Input: part model. Units: mm. Frame: model coordinates. A direction names the side the tool comes from. Round coordinates to 2 decimals unless told otherwise and drop trailing zeros. Order: outer loops, then holes, each group sorted by start corner. A loop starts at its lowest first (then second) coordinate and runs counter-clockwise, first axis right, second up.
Item 1: Reachability of faces 5 (the cylindrical face through (-2.75, 0.36, -12.4)), 6 (the flat face through (-6, -12, -44.45)) from +Z, -Z, +X, -X, +Y, -Y: full face, straight path, thin tool, end or side. Return the list, or none.
Item 2: Mould query, pull axis X, two halves, no side actions, for faces 1 (the flat face through (25.4, 0, -10)), 2 (the flat face through (-25.4, 0, -9)), 3 (the flat face through (-3, -6, -50.8)), 4 (the cylindrical face through (-1.03, -0.36, -20.75)). Classes: released by +X, released by -X, zero draft, split by the parting line, or undercut.
Item 3: Cut plane C-C on y = -7.5. Give the number of separate pieces and of enclosed holes in the cut face, then the cut area to 3 significant figures.
Item 4: Cut plane B-B on x = 8.5. Output: boundary loops of the cut face in (y, z).
Item 5: Cut plane A-A on z = -25.4. Output: boundary loops of the cut face in (x, y).
Item 6: Line query: L1, parallel to Z at x = 0, y = -1; L2, parallel to Z at x = 0, y = 9; L3, parallel to X at y = -10, z = -25. Output: solid intervals per line, ascending.
Item 7: First-contact query: pin 1 (4 mm diameter, centred on x = -1.5, y = 3, fed in from -Z); pin 2 (7.5 mm diameter, centred on x = 0, z = -25.4, fed in from +Y). Flat tips, straight axial feed; report the tip coordinate or a pass-through.
Item 8: Cut plane D-D on z = 0. Output: boundary loops of the cut face in (x, y).
```python
from build123d import *

# Parameters (mm, degrees)
F0_R     = 12.7
F1_DEPTH = 25.4


with BuildPart() as f1:
    # F0 (on Front) → F1 (new body, symmetric)
    with BuildSketch(Plane.XZ):
        Polygon((-12.7, -44.45), (0, -44.45), (12.7, -44.45), (25.4, -44.45), (25.4, 25.4), (-25.4, 25.4), (-25.4, -44.45), align=None)
        with BuildLine():
            ThreePointArc((0, -30.1625), (-3.3675960454, -22.0324039546), (4.7625, -25.4))
            ThreePointArc((4.7625, -25.4), (3.3675960454, -28.7675960454), (0, -30.1625))
        make_face(mode=Mode.SUBTRACT)
        Circle(F0_R, mode=Mode.SUBTRACT)
    extrude(amount=F1_DEPTH, both=True)

    # F0 (on Front) → F2 (revolve)
    with BuildSketch(Plane.XZ):
        Polygon((12.7, -44.45), (0, -44.45), (0, -50.8), (6.35, -50.8), (12.7, -50.8), align=None)
        Polygon((6.35, -50.8), (0, -50.8), (0, -53.34), (2.54, -53.34), (6.35, -53.34), align=None)
        Polygon((2.54, -53.34), (0, -53.34), (0, -57.15), align=None)
    revolve(axis=Axis((0, 0, -41.275), (0, 0, -1)))


solid = f1.part
```
From the geometry:
1. face 5: +Y, -Y
1. face 6: -Z
2. face 1: released by +X
2. face 2: released by -X
2. face 3: zero draft
2. face 4: undercut
3. separate pieces: 1
3. enclosed holes: 2
3. area: 3,100 mm2
4. outline: (-25.4, -44.45) - (-9.44, -44.45) - (-9.44, -50.8) - (9.44, -50.8) - (9.44, -44.45) - (25.4, -44.45) - (25.4, -9.44) - (-25.4, -9.44) - close; (-25.4, 9.44) - (25.4, 9.44) - (25.4, 25.4) - (-25.4, 25.4) - close
5. outline: (-25.4, -25.4) - (-4.76, -25.4) - (-4.76, 25.4) - (-25.4, 25.4) - close; (4.76, -25.4) - (25.4, -25.4) - (25.4, 25.4) - (4.76, 25.4) - close
6. L1: z = -55.65 to -30.16, -20.64 to -12.7, 12.7 to 25.4
6. L2: z = -50.8 to -30.16, -20.64 to -12.7, 12.7 to 25.4
6. L3: x = -25.4 to -4.75, 4.75 to 25.4
7. pin 1: stops at z = -55.12
7. pin 2: passes through
8. outline: (-25.4, -25.4) - (-12.7, -25.4) - (-12.7, 25.4) - (-25.4, 25.4) - close; (12.7, -25.4) - (25.4, -25.4) - (25.4, 25.4) - (12.7, 25.4) - close
